from build123d import *

# Parameters (mm, degrees)
ESBO_O1_W                = 42
ESBO_O1_H                = 6.5
RESSALTO_EXTRUS_O1_DEPTH = 3
ESBO_O2_R                = 1.5
CORTE_EXTRUS_O1_DEPTH    = 22.460719932
ESBO_O3_R                = 2.75
CORTE_EXTRUS_O2_DEPTH    = 2
FILETE1_R                = 3.25


with BuildPart() as part:
    # Esboço1 → Ressalto-extrusão1 (new body)
    with BuildSketch(Plane(origin=(0, 0, 0), x_dir=(1, 0, 0), z_dir=(0, 1, 0))):
        Rectangle(ESBO_O1_W, ESBO_O1_H)
    extrude(amount=RESSALTO_EXTRUS_O1_DEPTH)

    # Esboço2 → Corte-extrusão1 (cut, through all)
    with BuildSketch(Plane(origin=(0, 3, 0), x_dir=(1, 0, 0), z_dir=(0, 1, 0))):
        with Locations(Location((16, 0, 0), (0, 0, 270))):
            Circle(ESBO_O2_R)
        with BuildLine():
            Line((-16, 1.5), (-12, 1.5))
            ThreePointArc((-12, 1.5), (-10.5, 0), (-12, -1.5))
            Line((-12, -1.5), (-16, -1.5))
            ThreePointArc((-16, -1.5), (-17.5, 0), (-16, 1.5))
        make_face()
    extrude(amount=-CORTE_EXTRUS_O1_DEPTH, mode=Mode.SUBTRACT)

    # Esboço3 → Corte-extrusão2 (cut)
    with BuildSketch(Plane(origin=(0, 3, 0), x_dir=(1, 0, 0), z_dir=(0, 1, 0))):
        with Locations(Location((16, 0, 0), (0, 0, 270))):
            Circle(ESBO_O3_R)
        with BuildLine():
            Line((-16, 2.75), (-12, 2.75))
            ThreePointArc((-12, 2.75), (-9.25, 0), (-12, -2.75))
            Line((-12, -2.75), (-16, -2.75))
            ThreePointArc((-16, -2.75), (-18.75, 0), (-16, 2.75))
        make_face()
    extrude(amount=-CORTE_EXTRUS_O2_DEPTH, mode=Mode.SUBTRACT)

    # Filete1
    filete1_edges = [part.edges().sort_by_distance(p)[0] for p in [
        (21, 1.5, 3.25),
        (21, 1.5, -3.25),
        (-21, 1.5, 3.25),
        (-21, 1.5, -3.25),
    ]]
    fillet(filete1_edges, radius=FILETE1_R - 0.0001)  # a hair under: the kernel refuses the full size


solid = part.part
Can you work these out from the model? Positions are in its coordinate system, mm. A direction names the side the tool comes from. Give positions to 0.01 mm unless a question says otherwise; leave off trailing zeros. Loops run counter-clockwise (first coordinate to the right, second up) from the corner with the lowest first, then second, coordinate; pieces in that order, holes last. Notation, with made-up numbers: (-4, -36) -> (1, -36) arc R22 cw to (1, -25) -> close; hole circle Ø2 at (-19.5, -30). An arc over 180 degrees is marked (long way). Return JSON: item names as keys, results as strings.
Q1. I want a section at B-B, the plane y = 2.15. Count the separate pieces of the cut face and the enclosed holes in it, then the cut area to 3 significant figures.
Checks:
{"separate pieces": "1", "enclosed holes": "2", "area": "194 mm2"}
Q2. We'd pull the mould along X, two halves only. Please class faces 4 (the face through (-9.25, 2.01, -0.06)), 5 (the face through (0, 0, 0)), 6 (the face through (20.023, 1.521, -2.323)): released by +X, released by -X, zero draft, split by the parting line, or undercut.
Checks:
{"face 4": "undercut", "face 5": "zero draft", "face 6": "released by +X"}
Q3. On a 3-axis mill with a long thin cutter (end or side, diameter ignored), from which of +Z, -Z, +X, -X, +Y, -Y can I reach the whole of each face in a straight line? I mean faces 1 (the face through (-18.75, 2.01, 0.06)), 2 (the face through (-20.073, 1.521, 2.273)), 3 (the face through (-14, 0.5, 1.5)). Say none if no direction works.
Checks:
{"face 1": "+Y", "face 2": "+Z, -X, +Y, -Y", "face 3": "+Y, -Y"}
Q4. I need wall thicknesses on probe 1 along X at (y, z) = (0.75, 0); probe 2 along X at (y, z) = (2.65, 0); probe 3 along Z at (x, y) = (14.5, 1.6). Which ranges of each line are inside material? Lowest first, please.
Checks:
{"probe 1": "x = -21 to -17.5, -10.5 to 14.5, 17.5 to 21", "probe 2": "x = -21 to -18.75, -9.25 to 13.25, 18.75 to 21", "probe 3": "z = -3.25 to -2.3, 2.3 to 3.25"}
Q5. For pin 1 Ø1.5 at (y, z) = (0.5, 1) entering from +X; pin 2 Ø1.6 at (x, z) = (17, -0.5) entering from +Y, each with a flat end and sliding along its axis, tell me the tip position at first contact or that it passes through.
Checks:
{"pin 1": "stops at x = 20.99", "pin 2": "stops at y = 1"}
Q6. I want a section at C-C, the plane z = 2. List the corners of the cut face in (x, y) for me.
Checks:
{"outline": "(-20.31, 0) -> (20.31, 0) -> (20.31, 3) -> (17.89, 3) -> (17.89, 1) -> (14.11, 1) -> (14.11, 3) -> (-10.11, 3) -> (-10.11, 1) -> (-17.89, 1) -> (-17.89, 3) -> (-20.31, 3) -> close"}
Q7. I want a section at A-A, the plane x = 16. List the corners of the cut face in (y, z) for me.
Checks:
{"outline": "(0, -3.25) -> (3, -3.25) -> (3, -2.75) -> (1, -2.75) -> (1, -1.5) -> (0, -1.5) -> close; (0, 1.5) -> (1, 1.5) -> (1, 2.75) -> (3, 2.75) -> (3, 3.25) -> (0, 3.25) -> close"}
